Autodesk Inventor part; units mm, degrees
ref_plane "Work Plane1" through (3.3655, 6.35, 0) normal (0, 1, 0) x (-1, 0, 0)
ref_plane "YZ Plane" through (0, 0, 0) normal (1, 0, 0) x (0, 1, 0)
ref_plane "XZ Plane" through (0, 0, 0) normal (0, 1, 0) x (-1, 0, 0)
sketch "Sketch2" plane through (0, 0, 0) normal (0, 0, 1) x (1, 0, 0)
  line L0 (0, 0) -> (7.62, 0)
  line L1 (-0.4445, 6.35) -> (7.1755, 6.35)
  line L2 (7.1755, 6.35) -> (7.1755, 3.175)
  line L3 (7.1755, 3.175) -> (-0.4445, 3.175)
  line L4 (-0.4445, 3.175) -> (-0.4445, 6.35)
  point P0 (3.3655, 6.35)
  dimension "d8" = 7.62
  dimension "d9" = 3.175
  dimension "d10" = 7.62
  dimension "d11" = 3.175
revolve "Revolution1" add sketch "Sketch2" angle 360 about axis through (0, 0, 0) along (1, 0, 0)
ref_plane "Work Plane1" through (3.3655, 6.35, 0) normal (0, 1, 0) x (-1, 0, 0)
sketch "Sketch3" plane through (3.3655, 6.35, 0) normal (0, 1, 0) x (-1, 0, 0)
  point P0 (3.3655, 0)
  point P1 (0, 0)
hole "Hole1" at (3.3655, 6.35, 0) direction (0, -1, 0) diameter 3.9624 depth 3.175 tip angle 118
equation "\"d10\" = d8"
properties part number "Collar" material "Aluminum 6061"
The listing builds one solid part. Answer for the finished solid, in the listing's coordinates (mm). A direction names the side the tool comes from. Give positions to 0.01 mm unless a question says otherwise; leave off trailing zeros. Order: outer loops, then holes, each group sorted by start corner. A loop starts at its lowest first (then second) coordinate and runs counter-clockwise, first axis right, second up. Notation, with made-up numbers: (72, 40.5) -> (102, 40.5) arc R18 ccw to (102, 62.5) -> close; hole circle Ø8 at (-7, -8). An arc over 180 degrees is marked (long way). Answer as a JSON object with one key per item and string values. Group by question number.
Item 1: The part is cut by section C-C on z = -1. Give the number of separate pieces and of enclosed holes in the cut face, and give its area (3 significant figures).
Item 2: The part is cut by section B-B on x = 5.75. Write down the section's boundary in (y, z) (3 decimals), and give its area (3 significant figures).
Item 3: The part is cut by section D-D on y = -2.5. Write down the section's boundary in (x, z).
Item 4: A tool of negligible diameter and unlimited length cuts with its end or side. For faces 1 (the conical face through (3.4, 2.935, -1.581)), 2 (the cylindrical face through (3.31, -3.17, -0.14)), from which of +Z, -Z, +X, -X, +Y, -Y can it reach the whole face along a straight path? Write none if from no direction.
Item 5: Determine the mould class of faces 3 (the conical face through (3.331, 2.935, 1.581)), 4 (the cylindrical face through (3.42, -5.04, -3.86)), 5 (the flat face through (7.176, -2, 3)) for opening direction Z: pulls with the +Z half, pulls with the -Z half, needs draft (parallel to the pull), parting line crosses it, or undercut.
Item 6: Consider L1, parallel to Z at x = 2.5, y = 0 (3 decimals); L2, parallel to X at y = 4.25, z = 0; L3, parallel to Z at x = 2, y = 5.5. Determine where each line is inside the solid, lowest interval first. Write a range as from..to.
Result set:
{
 "1": {"separate pieces": "3", "enclosed holes": "0", "area": "38.6 mm²"},
 "2": {"outline": "circle Ø12.7 at (0, 0); hole circle Ø6.35 at (0, 0)", "area": "95.0 mm²"},
 "3": {"outline": "(-0.44, -5.84) -> (7.18, -5.84) -> (7.18, -1.96) -> (-0.44, -1.96) -> close; (-0.44, 1.96) -> (7.18, 1.96) -> (7.18, 5.84) -> (-0.44, 5.84) -> close"},
 "4": {"face 1": "+Y", "face 2": "+X, -X"},
 "5": {"face 3": "undercut", "face 4": "parting line crosses it", "face 5": "needs draft"},
 "6": {"L1": "-6.35..-3.175, 3.175..6.35", "L2": "-0.44..1.38, 5.35..7.18", "L3": "-3.17..-1.44, 1.44..3.17"}
}
